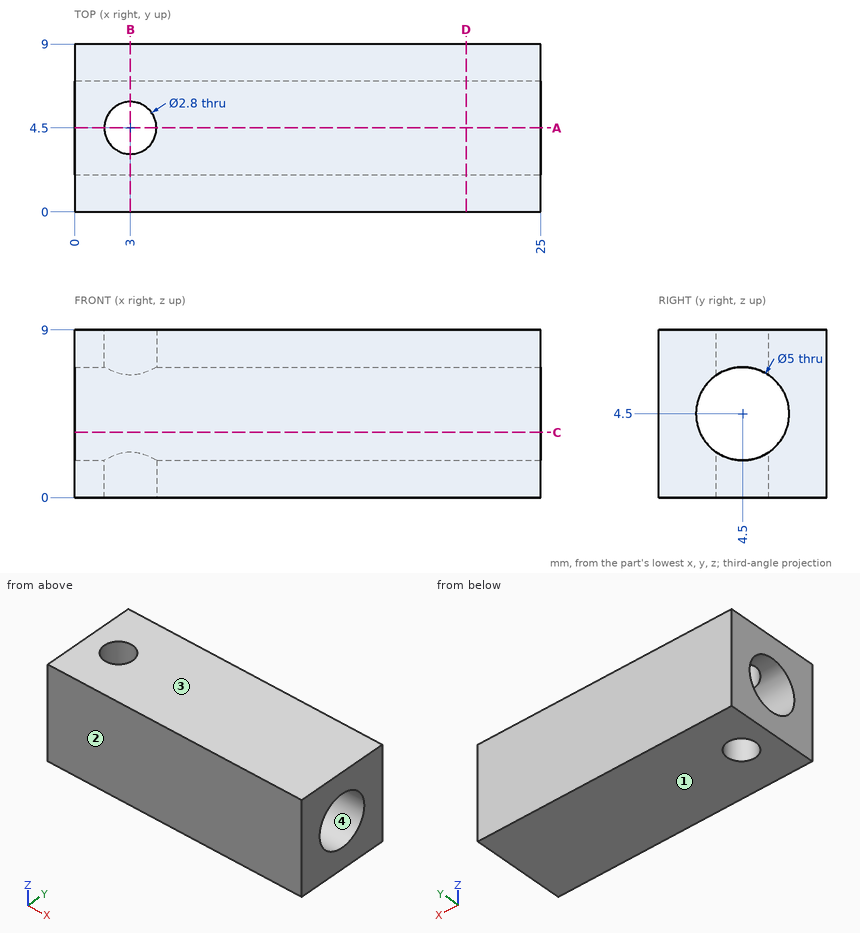
The figure shows three views and two pictorial views of one solid part (mm, origin at its lowest corner). Answer the questions. Round coordinates to 2 decimals unless told otherwise and drop trailing zeros. Write each loop counter-clockwise with the first axis right and the second up, starting at its lowest first coordinate (ties: lowest second). Pieces come first, ordered by that corner, then holes. Notation, with made-up numbers: (7, 21) -> (37, 21) arc R9 cw to (37, 35) -> close; hole circle Ø9 at (67.25, -3.75). An arc over 180 degrees is marked (long way). Answer as a JSON object with one key per item and string values. Group by question number.
Q1. Section B-B (x = 3) is taken. Write down the section's boundary in (y, z), plus the area to 3 significant figures.
Q2. Determine the mould class of the marked faces 1, 2, 3 and 4 for opening direction Z: pulls with the +Z half, pulls with the -Z half, needs draft (parallel to the pull), parting line crosses it, or undercut.
Q3. Straight lines are drawn through the part: line 1 along X through (y, z) = (4.5, 1.95); line 2 along Y through (x, z) = (3, 0.9); line 3 along Z through (x, y) = (18, 4.5). For each, find the intervals that lie inside material, in ascending order.
Q4. Section C-C (z = 3.5) is taken. Write down the section's boundary in (x, y), plus the area to 3 significant figures.
Q5. Section D-D (x = 21) is taken. Write down the section's boundary in (y, z).
Q6. Section A-A (y = 4.5) is taken. Write down the section's boundary in (x, z), plus the area to 3 significant figures.
Check values:
{
 "1": {"outline": "(0, 0) -> (3.1, 0) -> (3.1, 2.43) arc R2.5 cw to (3.1, 6.57) -> (3.1, 9) -> (0, 9) -> close; (5.9, 0) -> (9, 0) -> (9, 9) -> (5.9, 9) -> (5.9, 6.57) arc R2.5 cw to (5.9, 2.43) -> close", "area": "49.4 mm^2"},
 "2": {"face 1": "pulls with the -Z half", "face 2": "needs draft", "face 3": "pulls with the +Z half", "face 4": "undercut"},
 "3": {"line 1": "0 to 1.6, 4.4 to 25", "line 2": "0 to 3.1, 5.9 to 9", "line 3": "0 to 2, 7 to 9"},
 "4": {"outline": "(0, 0) -> (25, 0) -> (25, 2.21) -> (0, 2.21) -> close; (0, 6.79) -> (25, 6.79) -> (25, 9) -> (0, 9) -> close", "area": "110 mm^2"},
 "5": {"outline": "(0, 0) -> (9, 0) -> (9, 9) -> (0, 9) -> close; hole circle Ø5 at (4.5, 4.5)"},
 "6": {"outline": "(0, 0) -> (1.6, 0) -> (1.6, 2) -> (0, 2) -> close; (0, 7) -> (1.6, 7) -> (1.6, 9) -> (0, 9) -> close; (4.4, 0) -> (25, 0) -> (25, 2) -> (4.4, 2) -> close; (4.4, 7) -> (25, 7) -> (25, 9) -> (4.4, 9) -> close", "area": "88.8 mm^2"}
}
